For this review, take the finished solid that the model builds, in its own axes (mm). A direction names the side the tool comes from. Give positions to 0.01 mm unless a question says otherwise; leave off trailing zeros. Put each result on its own line as item: value.
from build123d import *

# Parameters (mm, degrees)
SKETCH2_R                = 7.5
BOSS_EXTRUDE1_DEPTH      = 25
SKETCH14_R               = 10.5
SKETCH14_R_2             = 10
EXTRUDE_THIN3_DEPTH      = 3
EXTRUDE_THIN3_DEPTH_BACK = 12
SKETCH8_R                = 10
CUT_EXTRUDE4_DEPTH       = 13
SKETCH12_R               = 10.5
SKETCH12_R_2             = 10
EXTRUDE_THIN2_DEPTH      = 12


with BuildPart() as part:
    # Sketch2 → Boss-Extrude1 (new body)
    with BuildSketch(Plane.XY):
        Polygon((0, 9.022413356), (-14.374271139, 4.248669099), (-8.495026865, -16.951200871), (8.495026865, -16.951200871), (14.374271139, 4.248669099), align=None)
        Circle(SKETCH2_R, mode=Mode.SUBTRACT)
    extrude(amount=-BOSS_EXTRUDE1_DEPTH)

    # Sketch14 → Extrude-Thin3 (add, two sides)
    with BuildSketch(Plane(origin=(-8.98162527, -2.490825133, 2.158943025), x_dir=(0.267238376, -0.963630453, 0), z_dir=(0.938775452, 0.260345474, -0.225656566))) as extrude_thin3_sk:
        with Locations((3.064496194, 15.047052931)):
            Circle(SKETCH14_R)
        with Locations((3.064496194, 15.047052931)):
            Circle(SKETCH14_R_2, mode=Mode.SUBTRACT)
    extrude(amount=EXTRUDE_THIN3_DEPTH)
    extrude(extrude_thin3_sk.sketch, amount=-EXTRUDE_THIN3_DEPTH_BACK)

    # Sketch8 → Cut-Extrude4 (cut)
    with BuildSketch(Plane(origin=(21.957149201, -6.089256391, 0), x_dir=(0, 0, -1), z_dir=(0.963630453, -0.267238376, 0))):
        with Locations((12.31580825, -2.819568794)):
            Circle(SKETCH8_R)
    extrude(amount=-CUT_EXTRUDE4_DEPTH, mode=Mode.SUBTRACT)

    # Sketch12 → Extrude-Thin2 (add)
    with BuildSketch(Plane(origin=(21.957149201, -6.089256391, 0), x_dir=(0, 0, -1), z_dir=(0.963630453, -0.267238376, 0))):
        with Locations((12.31580825, -2.819568794)):
            Circle(SKETCH12_R)
        with Locations((12.31580825, -2.819568794)):
            Circle(SKETCH12_R_2, mode=Mode.SUBTRACT)
    extrude(amount=-EXTRUDE_THIN2_DEPTH)


solid = part.part
1) For faces 1 (the face through (0, -16.951, -12)), 2 (the face through (-7.493, 0.33, -12.325)), 3 (the face through (0, -10, 0)), 4 (the face through (-11.47, -6.22, -12.36)), list the 3-axis set-ups (+Z, -Z, +X, -X, +Y, -Y) from which the entire face can be reached by the end or side of a thin tool; tool diameter is ignored.
Geometry check:
face 1: +Z, -Z, -Y
face 2: +Z, -Z
face 3: +Z, +X, +Y, -Y
face 4: none
2) Insertion check: pin 1 Ø10 at (x, z) = (16, -3.5) entering from +Y; pin 2 Ø5 at (y, z) = (2.5, -7.5) entering from -X; pin 3 Ø8.5 at (x, z) = (-4, -18) entering from -Y; pin 4 Ø12 at (x, y) = (17, 4) entering from -Z. Each pin has a flat end and moves straight along its axis. Give the tip position at first contact, or say it passes through.
Geometry check:
pin 1: stops at y = 5.37
pin 2: stops at x = -25.37
pin 3: stops at y = -16.95
pin 4: stops at z = -25
3) Draft analysis for pull direction X (two halves, no side actions). For faces 5 (the face through (0, -10, -25)), 6 (the face through (-7.087, 6.669, -12.325)), 7 (the face through (-9.516, -13.269, -3.992)), 8 (the face through (7.3, 6.6, -12.3)), state which applies: pulls with the +X half, pulls with the -X half, needs draft (parallel to the pull), parting line crosses it, or undercut.
Geometry check:
face 5: needs draft
face 6: pulls with the -X half
face 7: undercut
face 8: pulls with the +X half
4) Wall thickness on line 1 (Y direction, x = 0, z = -7.75); line 2 (Z direction, x = -10, y = -2); line 3 (Z direction, x = 14, y = -1.25): over which ranges is each line inside the solid? List them lowest first.
Geometry check:
line 1: y = -16.95 to -7.5, 7.5 to 9.02
line 2: z = -25 to 0
line 3: z = -21.35 to -20.76, -3.87 to -3.28
